Input: dimensioned drawing with shaded views. Units: mm. Origin: part minimum x, y, z. Give positions to 0.01 mm unless a question says otherwise; leave off trailing zeros. Loops run counter-clockwise (first coordinate to the right, second up) from the corner with the lowest first, then second, coordinate; pieces in that order, holes last.
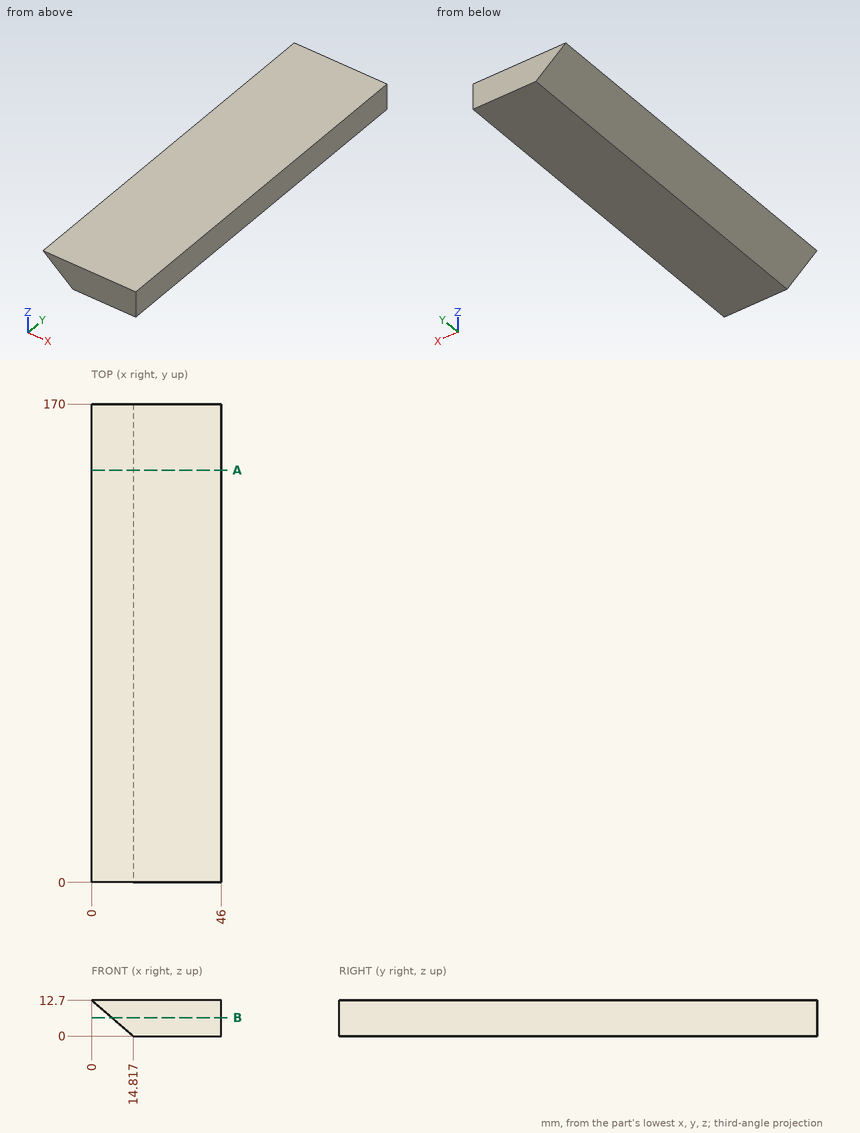
Item 1: Section query A-A on y = 146.5. Return loops of the section in (x, z), plus the area to 3 significant figures.
Values follow:
outline: (0, 12.7) - (14.82, 0) - (46, 0) - (46, 12.7) - close
area: 490 mm2
Item 2: Pin query (flat end, axial travel): pin 1 (6 mm diameter, centred on y = 66.5, z = 3.5, fed in from -X) (1 decimal). Return the tip coordinate at first contact, or that it passes through.
Values follow:
pin 1: stops at x = 7.2
Item 3: Ray query, probe 1 along X at (y, z) = (77, 9.5) (1 decimal); probe 2 along X at (y, z) = (159, 8.5); probe 3 along Z at (x, y) = (6.5, 125). Return the intervals inside material, ascending.
Values follow:
probe 1: x = 3.7 to 46
probe 2: x = 4.9 to 46
probe 3: z = 7.13 to 12.7
Item 4: Section query B-B on z = 6.5. Return loops of the section in (x, y), plus the area to 3 significant figures.
Values follow:
outline: (7.23, 0) - (46, 0) - (46, 170) - (7.23, 170) - close
area: 6,590 mm2
